For this review, use the dimensioned drawing (mm, ordinates from the lowest corner) and the shaded views. Round coordinates to 2 decimals unless told otherwise and drop trailing zeros. Write each loop counter-clockwise with the first axis right and the second up, starting at its lowest first coordinate (ties: lowest second). Pieces come first, ordered by that corner, then holes. Notation, with made-up numbers: (-36.5, -35) - (-17.5, -35) arc R8 cw to (-17.5, -20) - close; hole circle Ø4 at (-12.5, -12.5). An arc over 180 degrees is marked (long way). Write each question's results on one line, items separated by ' | '.
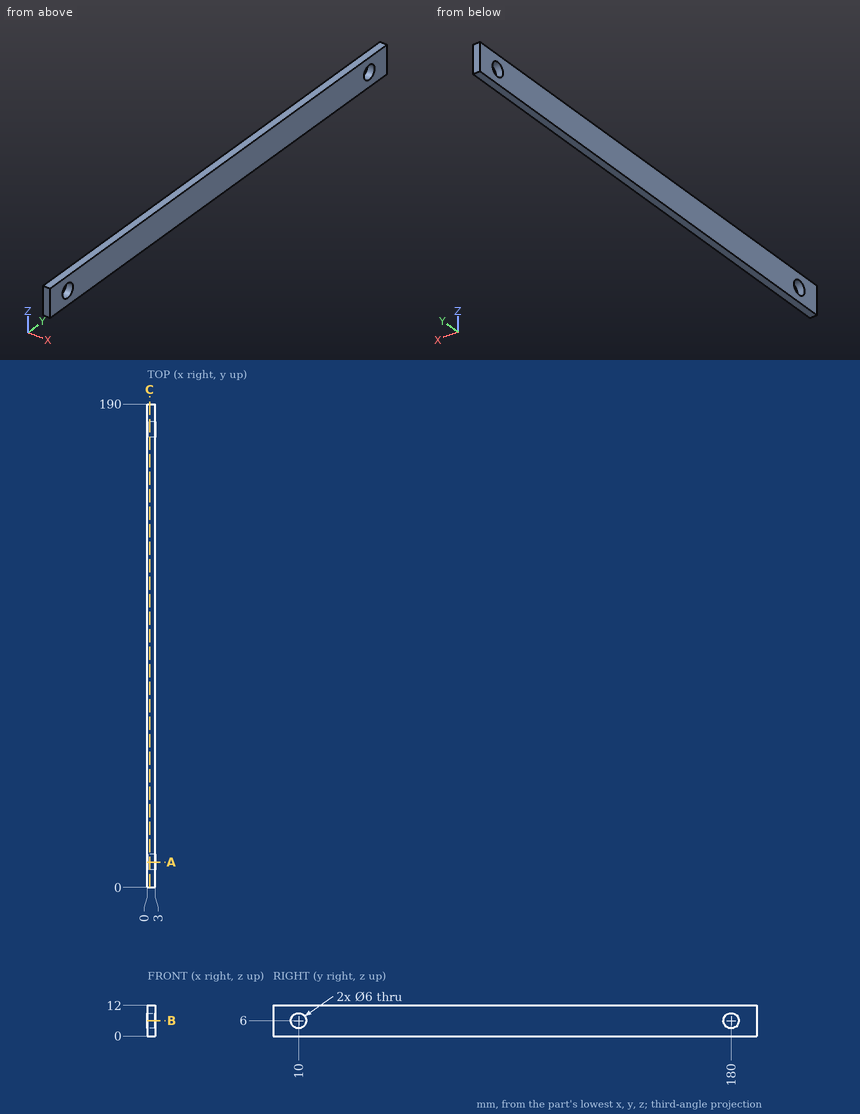
Q1. Insertion check: P1, Ø1.5, axis at y = 48.5, z = 10.5, coming from the -X side. The pin has a flat end and moves straight along its axis. Give the tip position at first contact, or say it passes through.
Evaluation:
P1: stops at x = 0
Q2. For probe 1 along Y at (x, z) = (1.8, 6); probe 2 along Z at (x, y) = (0.6, 180); probe 3 along Y at (x, z) = (0.6, 3.25), list the stretches that pass through material, from the lowest coordinate up.
Evaluation:
probe 1: y = 0 to 7, 13 to 177, 183 to 190 | probe 2: z = 0 to 3, 9 to 12 | probe 3: y = 0 to 8.8, 11.2 to 178.8, 181.2 to 190
Q3. We need section A-A (y = 10). State the section outline as (x, z) points, plus the area to 3 significant figures.
Evaluation:
outline: (0, 0) - (3, 0) - (3, 3) - (0, 3) - close; (0, 9) - (3, 9) - (3, 12) - (0, 12) - close | area: 18.0 mm^2
Q4. We need section B-B (z = 6). State the section outline as (x, y) points.
Evaluation:
outline: (0, 0) - (3, 0) - (3, 7) - (0, 7) - close; (0, 13) - (3, 13) - (3, 177) - (0, 177) - close; (0, 183) - (3, 183) - (3, 190) - (0, 190) - close
Q5. We need section C-C (x = 0.9). State the section outline as (y, z) points.
Evaluation:
outline: (0, 0) - (190, 0) - (190, 12) - (0, 12) - close; hole circle Ø6 at (10, 6); hole circle Ø6 at (180, 6)
